Autodesk Inventor part; units mm, degrees
ref_plane "YZ Plane" through (0, 0, 0) normal (1, 0, 0) x (0, 1, 0)
ref_plane "XZ Plane" through (0, 0, 0) normal (0, 1, 0) x (-1, 0, 0)
ref_plane "XY Plane" through (0, 0, 0) normal (0, 0, 1) x (1, 0, 0)
sketch "Sketch1" plane through (0, 0, 0) normal (0, 0, 1) x (1, 0, 0)
  line L0 (10.1192, 6.6438) -> (35.5192, 6.6438)
  line L1 (35.5192, 6.6438) -> (35.5192, 0.2938)
  line L2 (35.5192, 0.2938) -> (10.1192, 0.2938)
  line L3 (10.1192, 0.2938) -> (10.1192, 6.6438)
  point P0 (0, 0)
  dimension "d0" = 25.4
  dimension "d1" = 6.35
extrude "Extrusion1" add sketch "Sketch1" along normal blind 237.8075
sketch "Sketch2" plane through (10.1192, 6.6438, 0) normal (0, 1, 0) x (1, 0, 0)
  line L0 (0, 0) -> (25.4, 0)
  line L1 (0, 0) -> (0, -237.8075)
  line L2 (25.4, -237.8075) -> (0, -237.8075)
  line L3 (25.4, 0) -> (25.4, -237.8075)
  line L4 (12.7, 0) -> (12.7, -237.8075) construction
  line L5 (25.4, -237.8075) -> (0, -237.8075) construction
  line L6 (0, 0) -> (0, -237.8075) construction
  line L7 (0, -167.1637) -> (25.4, -167.1637) construction
  line L8 (0, -70.6437) -> (25.4, -70.6437) construction
  line L9 (25.4, 0) -> (25.4, -237.8075) construction
  circle A0 centre (12.7, -70.6437) radius 3.175
  circle A1 centre (12.7, -167.1637) radius 3.175
  line L10 (32.1721, -167.1637) -> (32.1721, -237.8075) construction
  line L11 (29.604, -70.6437) -> (29.604, 0) construction
  point P0 (-10.1192, 0)
  dimension "d6" = 6.35
  dimension "d7" = 6.35
  dimension "d10" = 96.52
extrude "Extrusion2" cut sketch "Sketch2" against normal through all contours A0 | A1
sketch "Sketch3" plane through (10.1192, 0.2938, 0) normal (-1, 0, 0) x (0, 0, 1)
  line L0 (44.8421, -2.7964) -> (94.9957, -2.7964)
  line L1 (94.9957, -2.7964) -> (94.9957, 2.2087)
  line L2 (94.9957, 2.2087) -> (44.8421, 2.2087)
  line L3 (44.8421, 2.2087) -> (44.8421, -2.7964)
  point P0 (0, -0.2938)
extrude "Extrusion3" cut sketch "Sketch3" against normal through all
sketch "Sketch4" plane through (10.1192, 6.6438, 0) normal (0, 1, 0) x (1, 0, 0)
  line L0 (18.35, -38.735) -> (6.35, -38.735)
  line L1 (6.35, -102.735) -> (18.35, -102.735)
  line L2 (18.35, -38.735) -> (7.105, -38.735)
  line L3 (7.105, -38.735) -> (7.105, -29.21)
  line L4 (7.105, -29.21) -> (18.35, -29.21)
  line L5 (18.35, -29.21) -> (18.35, -38.735)
  line L6 (18.35, -102.735) -> (6.35, -102.735)
  line L7 (6.35, -102.735) -> (6.35, -112.26)
  line L8 (6.35, -112.26) -> (18.35, -112.26)
  line L9 (18.35, -112.26) -> (18.35, -102.735)
  point P0 (-10.1192, 0)
  dimension "d13" = 9.525
  dimension "d14" = 9.525
extrude "Extrusion4" add sketch "Sketch4" along normal blind 30.1625
chamfer "Chamfer1" distance 4.7625 angle 45 2 edges at (22.8467, 6.6438, 29.21) (22.4692, 6.6438, 112.26)
sketch "Sketch5" plane through (16.4692, 36.8063, 112.26) normal (0, 0, 1) x (1, 0, 0)
  circle A0 centre (6, -22.1625) radius 1.3525
  circle A1 centre (6, -6.1625) radius 1.3525
  point P0 (-16.4692, -36.8063)
extrude "Extrusion5" cut sketch "Sketch5" against normal through all
fillet "Fillet1" radius 6.35 4 edges at (16.4692, 36.8063, 107.4975) (28.4692, 36.8063, 107.4975) (17.2242, 36.8063, 33.9725) (28.4692, 36.8063, 33.9725)
chamfer "Chamfer2" distance 4.7625 angle 45 4 edges at (16.4692, 6.6438, 109.8788) (28.4692, 6.6438, 109.8788) (28.4692, 6.6438, 31.5913) (17.2242, 6.6438, 31.5913)
sketch "Sketch6" plane through (10.1192, 6.6438, 0) normal (0, 1, 0) x (1, 0, 0)
  line L0 (25.4, -237.8075) -> (0, -237.8075)
  line L1 (18.6927, -237.8075) -> (21.1555, -237.8075)
  line L2 (21.1555, -212.4075) -> (21.1555, -112.0518)
  line L3 (21.1555, -112.0518) -> (18.6927, -112.0518)
  line L4 (18.6927, -112.0518) -> (18.6927, -212.4075)
  line L5 (6.7073, -237.8075) -> (4.2445, -237.8075)
  line L6 (4.2445, -212.4075) -> (4.2445, -112.0518)
  line L7 (4.2445, -112.0518) -> (6.7073, -112.0518)
  line L8 (6.7073, -112.0518) -> (6.7073, -212.4075)
  line L9 (25.4, 0) -> (25.4, -237.8075)
  line L10 (0, 0) -> (0, -237.8075)
  line L11 (21.1555, -171.8415) -> (25.4, -171.8415)
  line L12 (4.2445, -171.8415) -> (0, -171.8415)
  line L13 (20.8665, -0.289) -> (18.4037, -0.289)
  line L14 (18.4037, -34.2615) -> (20.8665, -34.2615)
  line L15 (7.105, -29.21) -> (2.3425, -24.4475)
  line L16 (3.9555, -0.289) -> (6.4182, -0.289)
  line L17 (6.4182, -28.5232) -> (3.9555, -28.5232)
  line L18 (31.115, -212.4075) -> (-5.715, -212.4075)
  point P0 (-10.1192, 0)
  point P1 (21.1555, -225.1075)
  point P2 (18.6927, -225.1075)
  point P3 (6.7073, -225.1075)
  point P4 (4.2445, -225.1075)
extrude "Extrusion6" add sketch "Sketch6" along normal blind 4.7625 draft -20 contours L18 L4 L3 L2 | L18 L6 L7 L8
sketch "Sketch7" plane through (10.1192, 6.6438, 0) normal (0, 1, 0) x (1, 0, 0)
  line L0 (18.35, -90.5879) -> (18.35, -50.8821) construction
  line L1 (6.35, -50.8821) -> (6.35, -90.5879) construction
  line L2 (18.35, -99.735) -> (18.35, -41.735) construction
  line L3 (6.35, -99.735) -> (18.35, -99.735) construction
  line L4 (6.35, -41.735) -> (6.35, -99.735) construction
  line L5 (18.35, -41.735) -> (6.35, -41.735) construction
  circle A0 centre (12.35, -54.735) radius 1.3525 construction
  circle A1 centre (12.35, -62.735) radius 1.3525 construction
  circle A2 centre (12.35, -78.735) radius 1.3525 construction
  circle A3 centre (12.35, -86.735) radius 1.3525 construction
  line L6 (1.5875, -102.735) -> (23.1125, -102.735)
  line L7 (23.1125, -38.735) -> (2.3425, -38.735)
  line L8 (25.4, 0) -> (25.4, -44.8421)
  line L9 (18.35, -102.735) -> (25.4, -102.735)
  line L10 (25.4, -102.735) -> (25.4, -38.735)
  line L11 (25.4, -38.735) -> (18.35, -38.735)
  line L12 (18.35, -38.735) -> (18.35, -102.735)
  line L13 (0, 0) -> (0, -237.8075)
  line L14 (0, -102.735) -> (6.35, -102.735)
  line L15 (6.35, -102.735) -> (6.35, -38.735)
  line L16 (6.35, -38.735) -> (0, -38.735)
  line L17 (0, -38.735) -> (0, -102.735)
  point P0 (-10.1192, 0)
extrude "Extrusion7" add sketch "Sketch7" along normal blind 3.175 contours L14 L13 L16 L7 L15 L6 | L12 L7 L11 L8 L10 L9 L6
sketch "Sketch8" plane through (35.5192, 6.6438, 38.735) normal (0, 0, -1) x (-1, 0, 0)
  line L0 (5.4625, 3.175) -> (2.2875, 0)
  line L1 (0, 3.175) -> (5.4625, 3.175)
  line L2 (0, 0) -> (0, 3.175)
  line L3 (2.2875, 0) -> (0, 0)
  line L4 (23.0575, 0) -> (19.8825, 3.175)
  line L5 (25.4, 0) -> (23.0575, 0)
  line L6 (25.4, 0) -> (25.4, 3.175)
  line L7 (19.8825, 3.175) -> (25.4, 3.175)
  point P0 (35.5192, -6.6438)
extrude "Extrusion8" cut sketch "Sketch8" against normal through all
properties part number "Top piece"
Part model, mm, in its own coordinate system. A direction names the side the tool comes from. Coordinates: 2 decimals unless noted, no trailing zeros. Loops run counter-clockwise (first coordinate to the right, second up) from the corner with the lowest first, then second, coordinate; pieces in that order, holes last. Notation, with made-up numbers: (85.25, 65) - (132.25, 65) arc R9 cw to (132.25, 74) - close; hole circle Ø7 at (38, 54). An arc over 180 degrees is marked (long way). Write item = value, one per line. Start each with the question number.
Item 1: Wall check: L1, parallel to Z at x = 23.25, y = 13 (3 decimals); L2, parallel to Z at x = 21.75, y = 5; L3, parallel to Y at x = 11.5, z = 60. Give the ranges that are in metal, low to high. Write a range as from..to.
Item 2: 3-axis set-ups, long thin cutter, end or side, ignore diameter. For faces 1 (the flat face through (26.4, 6.644, 70.3)), 2 (the flat face through (28.469, 21, 108)), 3 (the flat face through (22, 24, 112.26)), 4 (the flat face through (16.469, 21, 107)): which of +Z, -Z, +X, -X, +Y, -Y reach the whole face in a straight line?
Item 3: Cut at C-C, the plane z = 34. State how many separate pieces and enclosed holes the cut face has, and give its area (3 significant figures).
Item 4: Mould opens along X. For faces 5 (the cylindrical face through (22.406, 3.513, 164.016)), 6 (the flat face through (23, 0.294, 22)), 7 (the flat face through (28.469, 21, 34)) say: released by +X, released by -X, zero draft, split by the parting line, or undercut.
Item 5: Flat gauge pins, fed straight in: pin 1 Ø2 at (x, y) = (19, 28.5) entering from +Z; pin 2 Ø1.6 at (y, z) = (8, 86.5) entering from -X; pin 3 Ø5 at (x, z) = (22.82, 167.16) entering from -Y; pin 4 Ø9 at (x, y) = (23.5, 20) entering from -Z. Where does each tip first touch, or does it go through?
Item 6: Cut at B-B, the plane z = 80. Give the cut face in (x, y).
Item 7: Cut at A-A, the plane y = 22.5. Give the cut face in (x, z) (3 decimals), and give its area (3 significant figures).
Item 8: Cut at D-D, the plane y = 34. Give the cut face in (x, z) (3 decimals).
The answers:
q1.L1 = 29.21..38.735, 102.735..112.26
q1.L2 = 0..67.65, 73.63..164.17, 170.15..237.81
q1.L3 = 2.5..6.64
q2.face_1 = +Y
q2.face_2 = +Z, -Z, +X, +Y
q2.face_3 = +Z, +X, -X, +Y
q2.face_4 = +Z, -Z, -X, +Y
q3.separate_pieces = 1
q3.enclosed_holes = 2
q3.area = 495 mm2
q4.face_5 = undercut
q4.face_6 = zero draft
q4.face_7 = released by +X
q5.pin_1 = 112.26
q5.pin_2 = 13.02
q5.pin_3 = through
q5.pin_4 = 29.21
q6.outline = (10.12, 2.5) - (35.52, 2.5) - (35.52, 6.64) - (33.23, 6.64) - (30.06, 9.82) - (28.47, 9.82) - (28.47, 6.64) - (16.47, 6.64) - (16.47, 9.82) - (15.64, 9.82) - (12.46, 6.64) - (10.12, 6.64) - close
q7.outline = (16.469, 102.735) - (28.469, 102.735) - (28.469, 112.26) - (16.469, 112.26) - close; (17.224, 29.21) - (28.469, 29.21) - (28.469, 38.735) - (17.224, 38.735) - close
q7.area = 221 mm2
q8.outline = (17.55, 102.735) - (27.414, 102.735) - (27.414, 112.26) - (17.55, 112.26) - close; (18.305, 29.21) - (27.498, 29.21) - (27.498, 38.735) - (18.305, 38.735) - close
